Build history of the part. All positions in model axes, mm. A direction names the side the tool comes from. Round coordinates to 2 decimals unless told otherwise and drop trailing zeros. Order: outer loops, then holes, each group sorted by start corner. A loop starts at its lowest first (then second) coordinate and runs counter-clockwise, first axis right, second up. Notation, with made-up numbers: (5, -27.75) -> (38, -27.75) arc R25 ccw to (38, 0.25) -> close; hole circle Ø8 at (22, -11.5). An arc over 180 degrees is marked (long way). Answer as a JSON object with one key per item and string values.
from build123d import *

# Parameters (mm, degrees)
F1_DEPTH  = 40
F2_DEPTH  = 4
F3_DEPTH  = 3
F4_DEPTH  = 5
F6_DEPTH  = 4
F7_DEPTH  = 3
F8_DEPTH  = 5
F10_DEPTH = 2
F13_DEPTH = 50
F15_DEPTH = 1
F16_DEPTH = 50
F17_DEPTH = 40


# Not quite as in the source:
# - ends of sketch curves that miss each other by under 0.0002 mm in the source are joined


with BuildPart() as f1:
    # F0 (on Front) → F1 (new body)
    with BuildSketch(Plane.XZ):
        Polygon((-20, 38.838), (-25, 0), (-17.3563005304, 0), (-16.0689015912, 10), (-13.9011792574, 26.838), (-13, 33.838), (-13, 38.838), align=None)
        Polygon((-16.0689015912, 10), (-17.3563005304, 0), (17.3563005304, 0), (16.0689015912, 10), (0, 10), align=None)
        Polygon((-13.9011792574, 26.838), (-16.0689015912, 10), (0, 10), (16.0689015912, 10), (13.9011792574, 26.838), (-3.37943e-05, 26.838), align=None)
        Polygon((-13, 33.838), (-13.9011792574, 26.838), (3.37943e-05, 26.838), (13.9011792574, 26.838), (13, 33.838), (0, 33.838), align=None)
        Polygon((16.0689015912, 10), (17.3563005304, 0), (25, 0), (20, 38.838), (13, 38.838), (13, 33.838), (13.9011792574, 26.838), align=None)
    extrude(amount=F1_DEPTH)

    # F0 (on Front) → F2 (cut)
    with BuildSketch(Plane.XZ):
        Polygon((-13, 33.838), (-13.9011792574, 26.838), (3.37943e-05, 26.838), (13.9011792574, 26.838), (13, 33.838), (0, 33.838), align=None)
    extrude(amount=F2_DEPTH, mode=Mode.SUBTRACT)

    # F0 (on Front) → F3 (cut)
    with BuildSketch(Plane.XZ):
        Polygon((-16.0689015912, 10), (-17.3563005304, 0), (17.3563005304, 0), (16.0689015912, 10), (0, 10), align=None)
    extrude(amount=F3_DEPTH, mode=Mode.SUBTRACT)

    # F0 (on Front) → F4 (cut)
    with BuildSketch(Plane.XZ):
        Polygon((-13.9011792574, 26.838), (-16.0689015912, 10), (0, 10), (16.0689015912, 10), (13.9011792574, 26.838), (-3.37943e-05, 26.838), align=None)
    extrude(amount=F4_DEPTH, mode=Mode.SUBTRACT)

    # F5 (on face) → F6 (cut)
    with BuildSketch(Plane.XZ.offset(40)):
        Polygon((-13, 33.838), (-13.9011792574, 26.838), (3.37943e-05, 26.838), (13.9011792574, 26.838), (13, 33.838), (0, 33.838), align=None)
    extrude(amount=-F6_DEPTH, mode=Mode.SUBTRACT)

    # F5 (on face) → F7 (cut)
    with BuildSketch(Plane.XZ.offset(40)):
        Polygon((-16.0689015912, 10), (-17.3563005304, 0), (17.3563005304, 0), (16.0689015912, 10), (0, 10), align=None)
    extrude(amount=-F7_DEPTH, mode=Mode.SUBTRACT)

    # F5 (on face) → F8 (cut)
    with BuildSketch(Plane.XZ.offset(40)):
        Polygon((-13.9011792574, 26.838), (-16.0689015912, 10), (0, 10), (16.0689015912, 10), (13.9011792574, 26.838), (-3.37943e-05, 26.838), align=None)
    extrude(amount=-F8_DEPTH, mode=Mode.SUBTRACT)

    # F9 (on face) → F10 (join)
    with BuildSketch(Plane.XY.offset(33.838)):
        with BuildLine():
            ThreePointArc((-10, -28), (-9.4142135624, -29.4142135624), (-8, -30))
            Line((-8, -30), (8, -30))
            ThreePointArc((8, -30), (9.4142135624, -29.4142135624), (10, -28))
            Line((10, -28), (10, -12))
            ThreePointArc((10, -12), (9.4142135624, -10.5857864376), (8, -10))
            Line((8, -10), (-8, -10))
            ThreePointArc((-8, -10), (-9.4142135624, -10.5857864376), (-10, -12))
            Line((-10, -12), (-10, -28))
        make_face()
    extrude(amount=F10_DEPTH)

    # F12 (on face) → F13 (cut)
    with BuildSketch(Plane.YZ.offset(-25)):
        Polygon((-3, 38.838), (0, 0), (0, 38.838), align=None)
        Polygon((-40, 38.838), (-40, 0), (-37, 38.838), align=None)
    extrude(amount=F13_DEPTH, mode=Mode.SUBTRACT)

    # F14 (on face) → F15 (join)
    with BuildSketch(Plane.XY.offset(35.838)):
        Polygon((-7.9011683363, -13.2460867956), (-6.8714413478, -12.5374526663), (-6.9702730115, -11.2913658707), (-8.0988316637, -10.7539132044), (-9.1285586522, -11.4625473337), (-9.0297269885, -12.7086341293), align=None)
        Polygon((6.9702730115, -11.2913658707), (6.8714413478, -12.5374526663), (7.9011683363, -13.2460867956), (9.0297269885, -12.7086341293), (9.1285586522, -11.4625473337), (8.0988316637, -10.7539132044), align=None)
        Polygon((7.9011683363, -26.7539132044), (6.8714413478, -27.4625473337), (6.9702730115, -28.7086341293), (8.0988316637, -29.2460867956), (9.1285586522, -28.5374526663), (9.0297269885, -27.2913658707), align=None)
        Polygon((-6.9702730115, -28.7086341293), (-6.8714413478, -27.4625473337), (-7.9011683363, -26.7539132044), (-9.0297269885, -27.2913658707), (-9.1285586522, -28.5374526663), (-8.0988316637, -29.2460867956), align=None)
    extrude(amount=F15_DEPTH)

    # F12 (on face) → F16 (join)
    with BuildSketch(Plane.YZ.offset(-25)):
        Polygon((-20, 33.838), (-30.3862196818, 33.838), (-32.2275606365, 10), (-20, 10), (-7.7724393635, 10), (-9.6137803182, 33.838), align=None)
    extrude(amount=F16_DEPTH)

    # F0 (on Front) → F17 (cut)
    with BuildSketch(Plane.XZ):
        Polygon((-25, 38.838), (-25, 10), (-21.2873989392, 38.838), align=None)
        Polygon((21.2873989392, 38.838), (25, 10), (25, 38.838), align=None)
    extrude(amount=F17_DEPTH, mode=Mode.SUBTRACT)


solid = f1.part
1) Cut at C-C, the plane z = 34.5. Give the cut face in (x, y), plus the area to 3 significant figures.
Checked values:
{"outline": "(-20.56, -37.34) -> (-13, -37.34) -> (-13, -2.66) -> (-20.56, -2.66) -> close; (-10, -28) arc R2 ccw to (-8, -30) -> (8, -30) arc R2 ccw to (10, -28) -> (10, -12) arc R2 ccw to (8, -10) -> (-8, -10) arc R2 ccw to (-10, -12) -> close; (13, -37.34) -> (20.56, -37.34) -> (20.56, -2.66) -> (13, -2.66) -> close", "area": "921 mm²"}
2) Cut at D-D, the plane x = 3.5. Give the cut face in (y, z), plus the area to 3 significant figures.
Checked values:
{"outline": "(-37, 0) -> (-3, 0) -> (-3, 10) -> (-5, 10) -> (-5, 26.84) -> (-4, 26.84) -> (-4, 33.84) -> (-10, 33.84) -> (-10, 35.84) -> (-30, 35.84) -> (-30, 33.84) -> (-36, 33.84) -> (-36, 26.84) -> (-35, 26.84) -> (-35, 10) -> (-37, 10) -> close", "area": "1,110 mm²"}
3) Which spindle directions (+Z, -Z, +X, -X, +Y, -Y) get a long thin tool onto all of the face, cutting with end or side? Do faces 3 (the face through (-13, -20, 36)), 4 (the face through (9.4, -29.43, 34.82)), 5 (the face through (0, -36, 10)). Say none if no direction does.
Checked values:
{"face 3": "+Z, +Y, -Y", "face 4": "+Z, -Y", "face 5": "-Y"}
4) Cut at B-B, the plane y = -6.5. Give the cut face in (x, z), plus the area to 3 significant figures.
Checked values:
{"outline": "(-25, 0) -> (25, 0) -> (20, 38.84) -> (13, 38.84) -> (13, 33.84) -> (-13, 33.84) -> (-13, 38.84) -> (-20, 38.84) -> close", "area": "1,620 mm²"}
5) Probe L1, parallel to Y at x = 1, z = 18; L2, parallel to Y at x = -13.5, z = 9.5; L3, parallel to X at y = -29, z = 34. List the from-to ranges inside material, lowest first. Write a range as from..to.
Checked values:
{"L1": "y = -35..-5", "L2": "y = -37..-3", "L3": "x = -20.62..-13, -9.73..9.73, 13..20.62"}
6) Pull direction X, two halves, no side cores. Call faces 1 (the face through (0, -36, 30)), 2 (the face through (21, -20, 33.838)): pulls with the +X half, pulls with the -X half, needs draft (parallel to the pull), parting line crosses it, or undercut.
Checked values:
{"face 1": "undercut", "face 2": "needs draft"}
7) Cut at A-A, the plane x = -11.5. Give the cut face in (y, z).
Checked values:
{"outline": "(-37, 0) -> (-3, 0) -> (-3, 10) -> (-5, 10) -> (-5, 26.84) -> (-4, 26.84) -> (-4, 33.84) -> (-36, 33.84) -> (-36, 26.84) -> (-35, 26.84) -> (-35, 10) -> (-37, 10) -> close"}
8) Flat gauge pins, fed straight in: pin 1 Ø2 at (x, z) = (3.5, 34.5) entering from -Y; pin 2 Ø1.5 at (y, z) = (-28, 25.5) entering from +X; pin 3 Ø0.6 at (x, y) = (3, -36.5) entering from +Z. Where does each tip first touch, or does it go through?
Checked values:
{"pin 1": "stops at y = -36", "pin 2": "stops at x = 23.1", "pin 3": "stops at z = 10"}
